Check sheet for the modelled part. Datum: model origin and axes. Units: mm. A direction names the side the tool comes from. Round coordinates to 2 decimals unless told otherwise and drop trailing zeros. Write each loop counter-clockwise with the first axis right and the second up, starting at its lowest first coordinate (ties: lowest second). Pieces come first, ordered by that corner, then holes.
Item 1: Cross-section at C-C on z = 1.35. Enter the section's corners in (x, y).
Item 2: Go/stop test with flat-tipped pins: pin 1 Ø1.5 at (y, z) = (4, 0.5) entering from -X; pin 2 Ø3 at (x, z) = (-2.5, 1.5) entering from +Y; pin 3 Ø1 at (y, z) = (-1, -2) entering from +X. Record where each tip stops, or that it passes through.
Item 3: Release check for a two-part mould opening along Y. For faces 1 (the cylindrical face through (2.83, -1.75, 1.26)), 2 (the cylindrical face through (1.08, -4.88, -2.01)), 3 (the flat face through (0, 0, -2.5)) record: +Y half, -Y half, draft (parallel to the pull), parting line (faces both ways), or undercut.
Item 4: Cross-section at D-D on z = -2. Enter the section's corners in (x, y), plus the area to 3 significant figures.
Item 5: Material ranges on line 1 (Y direction, x = 3, z = -0.15); line 2 (Y direction, x = 3.25, z = 2.1); line 3 (Y direction, x = -2, z = -0.15), recorded low to high.
Item 6: Cross-section at B-B on z = 0.7. Enter the section's corners in (x, y).
Item 7: Tool access check on faces 4 (the flat face through (-0.4, 0, 2.5)), 5 (the flat face through (3, -2, 2)), 6 (the cylindrical face through (-4, 0, 1)). Record the directions out of +Z, -Z, +X, -X, +Y, -Y that give a thin tool (end or side, any length) a straight path to the whole face; none if there is none.
from build123d import *

# Parameters (mm, degrees)
BOSS_EXTRUDE1_DEPTH      = 2.5
BOSS_EXTRUDE1_DEPTH_BACK = 2.5
SKETCH1_R                = 4
SKETCH2_W                = 8
SKETCH2_H                = 3
CUT_EXTRUDE1_DEPTH       = 3
CUT_EXTRUDE2_DEPTH       = 2
CUT_EXTRUDE2_DEPTH_BACK  = 2
SKETCH3_R                = 2.5
CHAMFER1_SIZE            = 0.5
SKETCH4_R                = 5
BOSS_EXTRUDE2_DEPTH      = 1.5
CHAMFER2_SIZE            = 0.5
CHAMFER3_SIZE            = 0.5


with BuildPart() as part:
    # Sketch1 → Boss-Extrude1 (new, two sides: drawn at the far end of the back side and taken through both)
    with BuildSketch(Plane.XY.offset(-BOSS_EXTRUDE1_DEPTH_BACK)):
        Circle(SKETCH1_R)
    extrude(amount=BOSS_EXTRUDE1_DEPTH + BOSS_EXTRUDE1_DEPTH_BACK)

    # Sketch2 → Cut-Extrude1 (cut)
    with BuildSketch(Plane.XY.offset(2.5)):
        with Locations((4, 0)):
            Rectangle(SKETCH2_W, SKETCH2_H)
    extrude(amount=-CUT_EXTRUDE1_DEPTH, mode=Mode.SUBTRACT)

    # Sketch3 → Cut-Extrude2 (cut, two sides: drawn at the far end of the back side and taken through both)
    with BuildSketch(Plane(origin=(0, 0, 0), x_dir=(1, 0, 0), z_dir=(0, 1, 0)).offset(-CUT_EXTRUDE2_DEPTH_BACK)):
        with Locations((5, -2.5)):
            Circle(SKETCH3_R)
    extrude(amount=CUT_EXTRUDE2_DEPTH + CUT_EXTRUDE2_DEPTH_BACK, mode=Mode.SUBTRACT)

    # Chamfer1
    chamfer1_edges = [part.edges().sort_by_distance(p)[0] for p in [
        (-4, 0, 2.5),
    ]]
    chamfer(chamfer1_edges, length=CHAMFER1_SIZE)

    # Sketch4 → Boss-Extrude2 (add)
    with BuildSketch(Plane(origin=(0, 0, -2.5), x_dir=(-1, 0, 0), z_dir=(0, 0, -1))):
        Circle(SKETCH4_R)
    extrude(amount=-BOSS_EXTRUDE2_DEPTH)

    # Chamfer2
    chamfer2_edges = [part.edges().sort_by_distance(p)[0] for p in [
        (-4, 0, -1),
    ]]
    chamfer(chamfer2_edges, length=CHAMFER2_SIZE - 0.0001)  # a hair under: the kernel refuses the full size

    # Chamfer3
    chamfer3_edges = [part.edges().sort_by_distance(p)[0] for p in [
        (5, 0, -1),
    ]]
    chamfer(chamfer3_edges, length=CHAMFER3_SIZE)


solid = part.part
Response values:
1. outline: (0, -1.5) - (0, 1.5) - (2.78, 1.5) - (2.78, 2) - (3.46, 2) arc R4 ccw (long way) to (3.46, -2) - (2.78, -2) - (2.78, -1.5) - close
2. pin 1: stops at x = -2.33
2. pin 2: stops at y = 3.87
2. pin 3: stops at x = 4.97
3. face 1: undercut
3. face 2: parting line
3. face 3: draft
4. outline: circle Ø10 at (0, 0)
4. area: 78.5 mm2
5. line 1: y = -2.65 to -1.5, 1.5 to 2.65
5. line 2: y = -2.16 to -2, 2 to 2.16
5. line 3: y = -3.46 to 3.46
6. outline: (0, -1.5) - (0, 1.5) - (3.27, 1.5) - (3.27, 2) - (3.46, 2) arc R4 ccw (long way) to (3.46, -2) - (3.27, -2) - (3.27, -1.5) - close
7. face 4: +Z, +X, -X, +Y, -Y
7. face 5: +Z, +X
7. face 6: +Z
